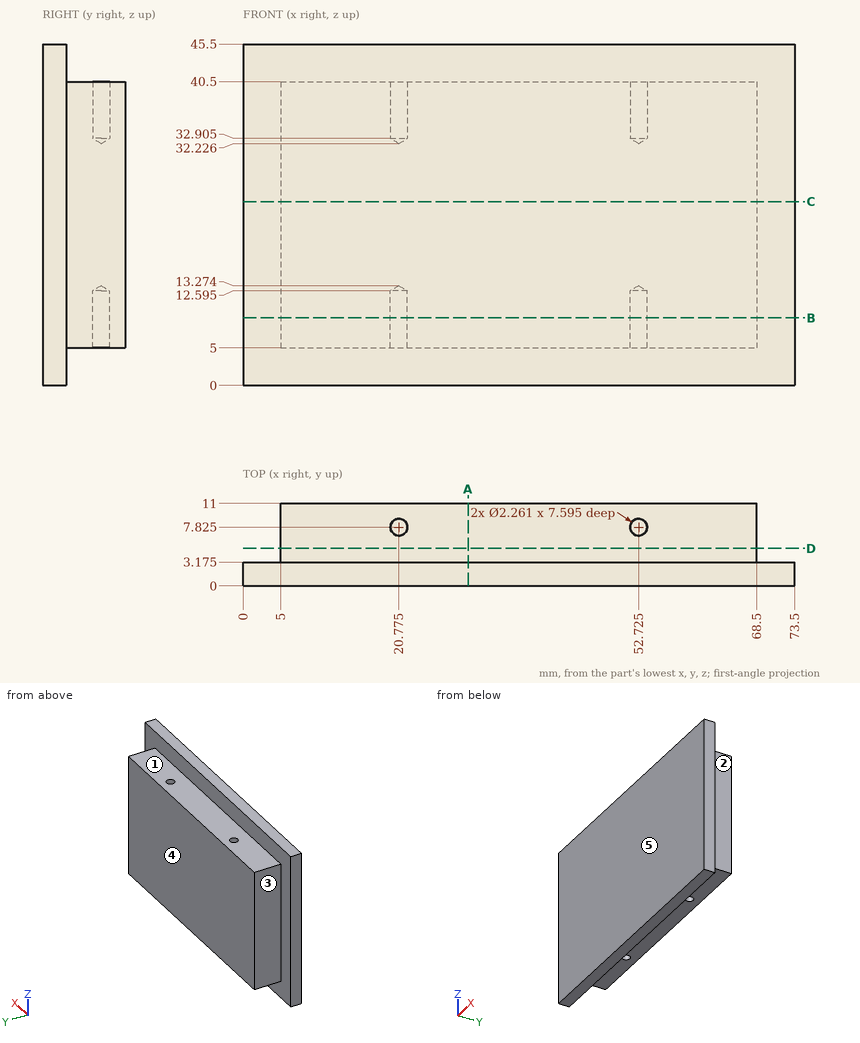
Part print with two shaded views. Sizes in mm from the minimum x, y, z corner. A direction names the side the tool comes from. Round coordinates to 2 decimals unless told otherwise and drop trailing zeros. Order: outer loops, then holes, each group sorted by start corner. A loop starts at its lowest first (then second) coordinate and runs counter-clockwise, first axis right, second up. Notation, with made-up numbers: (41.25, 76) -> (99.25, 76) arc R21 cw to (99.25, 106) -> close; hole circle Ø9 at (43.5, -35.5). An arc over 180 degrees is marked (long way). Write each question's results on one line, items separated by ' | '.
1. Cut at B-B (z = 9). Give the cut face in (x, y) (1 decimal).
Findings below:
outline: (0, 0) -> (73.5, 0) -> (73.5, 3.2) -> (68.5, 3.2) -> (68.5, 11) -> (5, 11) -> (5, 3.2) -> (0, 3.2) -> close; hole circle Ø2.3 at (20.8, 7.8); hole circle Ø2.3 at (52.7, 7.8)
2. 3-axis set-ups, long thin cutter, end or side, ignore diameter. For the marked faces 1, 2, 3, 4 and 5: which of +Z, -Z, +X, -X, +Y, -Y reach the whole face in a straight line?
Findings below:
face 1: +Z, +X, -X, +Y | face 2: +Z, -Z, +X, +Y | face 3: +Z, -Z, -X, +Y | face 4: +Z, -Z, +X, -X, +Y | face 5: +Z, -Z, +X, -X, -Y
3. Wall check: line 1 along Z through (x, y) = (65, 10.5); line 2 along X through (y, z) = (5, 34). Give the ranges that are in metal, low to high. Write a range as [from, to].
Findings below:
line 1: z = [5, 40.5] | line 2: x = [5, 68.5]
4. Flat gauge pins, fed straight in: P1, Ø1.4, axis at x = 20.775, y = 7.825, coming from the -Z side; P2, Ø2.5, axis at y = 6.5, z = 24, coming from the +X side; P3, Ø1, axis at x = 26.5, y = 4.5, coming from the -Z side. Where does each tip first touch, or does it go through?
Findings below:
P1: stops at z = 12.85 | P2: stops at x = 68.5 | P3: stops at z = 5
5. Cut at C-C (z = 24.5). Give the cut face in (x, y) (1 decimal), plus the area to 3 significant figures.
Findings below:
outline: (0, 0) -> (73.5, 0) -> (73.5, 3.2) -> (68.5, 3.2) -> (68.5, 11) -> (5, 11) -> (5, 3.2) -> (0, 3.2) -> close | area: 730 mm²
6. Cut at A-A (x = 30). Give the cut face in (y, z) (1 decimal).
Findings below:
outline: (0, 0) -> (3.2, 0) -> (3.2, 5) -> (11, 5) -> (11, 40.5) -> (3.2, 40.5) -> (3.2, 45.5) -> (0, 45.5) -> close
7. Cut at D-D (y = 5). Give the cut face in (x, z).
Findings below:
outline: (5, 5) -> (68.5, 5) -> (68.5, 40.5) -> (5, 40.5) -> close
